Geometry: final body of the model. Coordinates: model frame, mm. Round coordinates to 2 decimals unless told otherwise and drop trailing zeros. Loops run counter-clockwise (first coordinate to the right, second up) from the corner with the lowest first, then second, coordinate; pieces in that order, holes last. Notation, with made-up numbers: M 5,-33.75 L 27,-33.75 A16 ccw 27,-4.75 Z; hole C -29,43.5 d7. An arc over 180 degrees is marked long. Answer as a JSON object with one key per item and string values.
from build123d import *

# Parameters (mm, degrees)
CROQUIS1_R              = 1.5875
SALIENTE_EXTRUIR1_DEPTH = 3.175
CORTAR_EXTRUIR1_DEPTH   = 3.175
CORTAR_EXTRUIR3_DEPTH   = 10
CROQUIS5_R              = 10
CORTAR_EXTRUIR8_DEPTH   = 10
REDONDEO2_R             = 2
ESQUISSE1_RX            = 14
ESQUISSE1_RY            = 7
ENL_V_MAT_EXTRU_1_DEPTH = 43.027736377
ESQUISSE2_W             = 6.812613354
ESQUISSE2_H             = 3.3
ENL_V_MAT_EXTRU_2_DEPTH = 43.027736555


with BuildPart() as part:
    # Croquis1 → Saliente-Extruir1 (new body)
    with BuildSketch(Plane(origin=(0, 0, 0), x_dir=(1, 0, 0), z_dir=(0, 1, 0))):
        with BuildLine():
            Line((-12.5, 0), (-12.5, -40))
            Line((-12.5, -40), (-2.975, -40))
            Line((-2.975, -40), (-2.975, -20))
            ThreePointArc((-2.975, -20), (-0.046067812, -12.928932188), (7.025, -10))
            Line((7.025, -10), (12.5, -10))
            Line((12.5, -10), (12.5, 40))
            Line((12.5, 40), (2.5, 40))
            Line((2.5, 40), (-12.5, 0))
        make_face()
        with Locations(Location((-7.7375, -5, 0), (0, 0, 270))):
            Circle(CROQUIS1_R, mode=Mode.SUBTRACT)
        with Locations(Location((-7.7375, -35, 0), (0, 0, 270))):
            Circle(CROQUIS1_R, mode=Mode.SUBTRACT)
    extrude(amount=SALIENTE_EXTRUIR1_DEPTH)

    # Croquis2 → Cortar-Extruir1 (cut)
    with BuildSketch(Plane(origin=(0, 3.175, 0), x_dir=(1, 0, 0), z_dir=(0, 1, 0))):
        Polygon((12.5, -10), (6.1, 40), (12.5, 40), align=None)
    extrude(amount=-CORTAR_EXTRUIR1_DEPTH, mode=Mode.SUBTRACT)

    # Croquis3 → Cortar-Extruir3 (cut)
    with BuildSketch(Plane(origin=(0, 3.175, 0), x_dir=(1, 0, 0), z_dir=(0, 1, 0))):
        with BuildLine():
            ThreePointArc((-5.975, -30.575635639), (-7.7375, -30.2375), (-9.5, -30.575635639))
            Line((-9.5, -30.575635639), (-9.5, -9.427055314))
            ThreePointArc((-9.5, -9.427055314), (-7.7375, -9.765), (-5.975, -9.427055314))
            Line((-5.975, -9.427055314), (-5.975, -14.803847577))
            Line((-5.975, -14.803847577), (-5.975, -30.575635639))
        make_face()
        with BuildLine():
            ThreePointArc((-12.5, -35), (-7.7375, -39.7625), (-2.975, -35))
            Line((-2.975, -35), (-2.975, -40))
            Line((-2.975, -40), (-12.5, -40))
            Line((-12.5, -40), (-12.5, -35))
        make_face()
    extrude(amount=-CORTAR_EXTRUIR3_DEPTH, mode=Mode.SUBTRACT)

    # Croquis5 → Cortar-Extruir8 (cut)
    with BuildSketch(Plane(origin=(0, 3.175, 0), x_dir=(1, 0, 0), z_dir=(0, 1, 0))):
        with Locations((9.3, 15)):
            Circle(CROQUIS5_R)
        Polygon((7.025, -10), (11.878723404, -5.146276596), (12.5, -10), align=None)
    extrude(amount=-CORTAR_EXTRUIR8_DEPTH, mode=Mode.SUBTRACT)

    # Redondeo2
    redondeo2_edges = [part.edges().sort_by_distance(p)[0] for p in [
        (8.030358645, 1.5875, -24.919073083),
        (10.569641355, 1.5875, -5.080926917),
    ]]
    fillet(redondeo2_edges, radius=REDONDEO2_R)

    # Esquisse1 → Enlèv. mat.-Extru.1 (cut, through all)
    with BuildSketch(Plane(origin=(0, 3.175, 0), x_dir=(1, 0, 0), z_dir=(0, 1, 0))):
        with Locations(Location((6.096336345, 15.099252248), (0, 0, -90))):
            Ellipse(ESQUISSE1_RX, ESQUISSE1_RY)
    extrude(amount=-ENL_V_MAT_EXTRU_1_DEPTH, mode=Mode.SUBTRACT)

    # Esquisse2 → Enlèv. mat.-Extru.2 (cut, through all)
    with BuildSketch(Plane(origin=(0, 3.175, 0), x_dir=(1, 0, 0), z_dir=(0, 1, 0))):
        with Locations((11.483320122, 3.411473453)):
            Rectangle(ESQUISSE2_W, ESQUISSE2_H)
    extrude(amount=-ENL_V_MAT_EXTRU_2_DEPTH, mode=Mode.SUBTRACT)

    # Chanfrein1
    # the kernel refuses this chamfer: 5, 3.65932295 mm, written as the material it takes off along each edge
    with BuildSketch(Plane(origin=(7.533468678, -8.470907308, -28.801025952), x_dir=(-0.009849351174311172, 0, -0.9999514939643048), z_dir=(0, 1, 0))) as chanfrein1_piece_1:
        with BuildLine():
            Line((1.589139403, 0), (-0.217570658, 3.381370478))
            Line((-0.217570658, 3.381370478), (-0.306685884, 3.336000041))
            ThreePointArc((-0.306685884, 3.336000041), (0.203744233, 1.713157434), (-0.091827617, 0.03959405))
            Line((-0.091827617, 0.03959405), (0.011718833, -0.099310971))
            ThreePointArc((0.011718833, -0.099310971), (0.795376625, -0.006838256), (1.600858236, -0.099310971))
            Line((1.600858236, -0.099310971), (1.589139403, 0))
        make_face()
    extrude(amount=20.116814349, mode=Mode.SUBTRACT)


solid = part.part
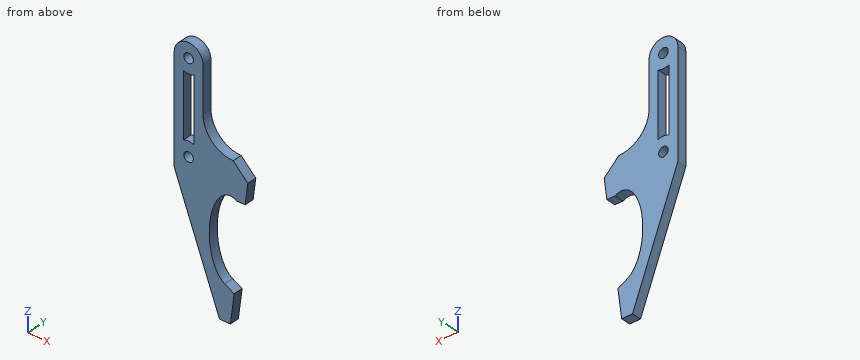
1) Section query D-D (x = 9.25). Return the cut outline in (y, z) (3 decimals).
Results:
{"outline": "M 0,-1.761 L 3.175,-1.761 L 3.175,7.775 L 0,7.775 Z"}
2) Section query B-B (y = 1.3). Count the separate pieces of the cut face and the enclosed holes in it, and give its area (3 significant figures).
Results:
{"separate pieces": "1", "enclosed holes": "3", "area": "741 mm2"}
3) Section query A-A (z = 13). Return the cut outline in (x, y) (3 decimals).
Results:
{"outline": "M -12.5,0 L -9.5,0 L -9.5,3.175 L -12.5,3.175 Z; M -5.975,0 L -0.116,0 L -0.116,3.175 L -5.975,3.175 Z"}
4) Pin query (flat end, axial travel): P1, Ø1, axis at x = -1.5, y = 0.5, coming from the +Z side; P2, Ø1.5, axis at x = 3, y = 3, coming from the +Z side; P3, Ø1, axis at y = 2, z = -14.5, coming from the -X side; P4, Ø3, axis at x = -7.74, z = 35, coming from the -Y side. Return the tip coordinate at first contact, or that it passes through.
Results:
{"P1": "z = 15.69", "P2": "z = 11.21", "P3": "x = -7.25", "P4": "through"}
5) Ray query, line 1 (X direction, y = 1.8, z = 35) (3 decimals); line 2 (X direction, y = 1.6, z = 21) (3 decimals); line 3 (Z direction, x = 10, y = 1.25) (3 decimals). Return the intervals inside material, ascending.
Results:
{"line 1": "-12.5 to -9.325, -6.15 to -2.975", "line 2": "-12.5 to -9.5, -5.975 to -2.975", "line 3": "-1.761 to 7.025"}
6) Section query C-C (z = 31.5). Return the cut outline in (x, y) (3 decimals), and give its area (3 significant figures).
Results:
{"outline": "M -12.5,0 L -2.975,0 L -2.975,3.175 L -12.5,3.175 Z", "area": "30.2 mm2"}
